The listing builds one solid part. Answer for the finished solid, in the listing's coordinates (mm). Coordinates: 2 decimals unless noted, no trailing zeros. Order: outer loops, then holes, each group sorted by start corner. A loop starts at its lowest first (then second) coordinate and runs counter-clockwise, first axis right, second up.
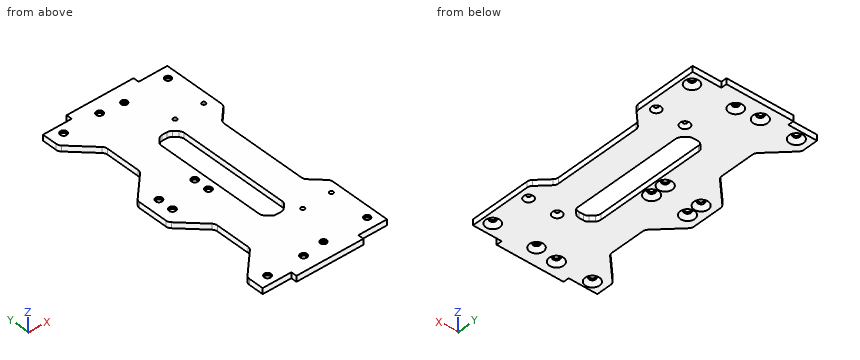
from build123d import *

# Parameters (mm, degrees)
SKETCH_1_W          = 65
SKETCH_1_H          = 129
SKETCH_1_W_2        = 35
SKETCH_1_H_2        = 6
EXTRUDE_1_DEPTH     = 3
SKETCH_2_R          = 1.75
CUT_EXTRUDE_1_DEPTH = 10
CHAMFER_1_SIZE      = 2
SKETCH_3_R          = 1
CUT_EXTRUDE_2_DEPTH = 10
CHAMFER_2_SIZE      = 1.5
CUT_EXTRUDE_3_DEPTH = 10
FILLET_1_R          = 3
CUT_EXTRUDE_4_DEPTH = 22
FILLET_2_R          = 3
SKETCH_6_R          = 1.625
CUT_EXTRUDE_5_DEPTH = 22
CHAMFER_3_SIZE      = 2
CUT_EXTRUDE_6_DEPTH = 22
FILLET_3_R          = 3


with BuildPart() as part:
    # Эскиз1 → Бобышка-Вытянуть1 (new body)
    with BuildSketch(Plane.XY):
        Rectangle(SKETCH_1_W, SKETCH_1_H)
        with Locations((0, 64.5)):
            Rectangle(SKETCH_1_W_2, SKETCH_1_H_2)
        with Locations((0, -64.5)):
            Rectangle(SKETCH_1_W_2, SKETCH_1_H_2)
    extrude(amount=EXTRUDE_1_DEPTH)

    # Эскиз2 → Вырез-Вытянуть1 (cut)
    with BuildSketch(Plane.XY.offset(3)):
        with Locations((-25.8, 59.9)):
            Circle(SKETCH_2_R)
        with Locations((-7, 59.9)):
            Circle(SKETCH_2_R)
        with Locations((-25.8, 4)):
            Circle(SKETCH_2_R)
        with Locations((-7, 4)):
            Circle(SKETCH_2_R)
        with Locations((-7, -4)):
            Circle(SKETCH_2_R)
        with Locations((-25.8, -4)):
            Circle(SKETCH_2_R)
        with Locations((-7, -59.9)):
            Circle(SKETCH_2_R)
        with Locations((-25.8, -59.9)):
            Circle(SKETCH_2_R)
    extrude(amount=-CUT_EXTRUDE_1_DEPTH, mode=Mode.SUBTRACT)

    # Фаска1
    chamfer_1_edges = [part.edges().sort_by_distance(p)[0] for p in [
        (-8.75, 4, 0),
        (-27.55, 4, 0),
        (-8.75, -4, 0),
        (-8.75, 59.9, 0),
        (-27.55, -59.9, 0),
        (-8.75, -59.9, 0),
        (-27.55, -4, 0),
        (-27.55, 59.9, 0),
    ]]
    chamfer(chamfer_1_edges, length=CHAMFER_1_SIZE)

    # Эскиз3 → Вырез-Вытянуть2 (cut)
    with BuildSketch(Plane(origin=(0, 0, 0), x_dir=(-1, 0, 0), z_dir=(0, 0, -1))):
        with Locations((-27.5, 37.5)):
            Circle(SKETCH_3_R)
        with Locations((-12.5, 37.5)):
            Circle(SKETCH_3_R)
        with Locations((-27.5, -37.5)):
            Circle(SKETCH_3_R)
        with Locations((-12.5, -37.5)):
            Circle(SKETCH_3_R)
    extrude(amount=-CUT_EXTRUDE_2_DEPTH, mode=Mode.SUBTRACT)

    # Фаска2
    chamfer_2_edges = [part.edges().sort_by_distance(p)[0] for p in [
        (13.5, 37.5, 0),
        (28.5, -37.5, 0),
        (13.5, -37.5, 0),
        (28.5, 37.5, 0),
    ]]
    chamfer(chamfer_2_edges, length=CHAMFER_2_SIZE)

    # Эскиз4 → Вырез-Вытянуть3 (cut)
    with BuildSketch(Plane(origin=(0, 0, 0), x_dir=(-1, 0, 0), z_dir=(0, 0, -1))):
        Polygon((32.5, 55.5), (19.5, 42.5), (19.5, 22), (32.5, 9), (37.771171481, 9), (37.771171481, 55.5), align=None)
        Polygon((37.771171481, -9), (32.5, -9), (19.5, -22), (19.5, -42.5), (32.5, -55.5), (37.771171481, -55.5), align=None)
    extrude(amount=-CUT_EXTRUDE_3_DEPTH, mode=Mode.SUBTRACT)

    # Скругление1
    fillet_1_edges = [part.edges().sort_by_distance(p)[0] for p in [
        (-32.5, 55.5, 1.5),
        (-32.5, 9, 1.5),
        (-19.5, 22, 1.5),
        (-19.5, 42.5, 1.5),
        (-32.5, -55.5, 1.5),
        (-19.5, -42.5, 1.5),
        (-19.5, -22, 1.5),
        (-32.5, -9, 1.5),
    ]]
    fillet(fillet_1_edges, radius=FILLET_1_R)

    # Эскиз5 → Вырез-Вытянуть4 (cut)
    with BuildSketch(Plane.XY.offset(3)):
        Polygon((1, 33.5), (6, 33.5), (9.5, 30), (9.5, -30), (6, -33.5), (1, -33.5), (-2.5, -30), (-2.5, 30), align=None)
    extrude(amount=-CUT_EXTRUDE_4_DEPTH, mode=Mode.SUBTRACT)

    # Скругление2
    fillet_2_edges = [part.edges().sort_by_distance(p)[0] for p in [
        (-2.5, 30, 1.5),
        (1, 33.5, 1.5),
        (6, 33.5, 1.5),
        (9.5, 30, 1.5),
        (9.5, -30, 1.5),
        (6, -33.5, 1.5),
        (1, -33.5, 1.5),
        (-2.5, -30, 1.5),
    ]]
    fillet(fillet_2_edges, radius=FILLET_2_R)

    # Эскиз6 → Вырез-Вытянуть5 (cut)
    with BuildSketch(Plane(origin=(0, 0, 0), x_dir=(-1, 0, 0), z_dir=(0, 0, -1))):
        with Locations((-27.5, 58.5)):
            Circle(SKETCH_6_R)
        with Locations((-4.64, 58.5)):
            Circle(SKETCH_6_R)
        with Locations(Location((-4.64, -58.5, 0), (0, 0, 180))):
            Circle(SKETCH_6_R)
        with Locations(Location((-27.5, -58.5, 0), (0, 0, 180))):
            Circle(SKETCH_6_R)
    extrude(amount=-CUT_EXTRUDE_5_DEPTH, mode=Mode.SUBTRACT)

    # Фаска3
    chamfer_3_edges = [part.edges().sort_by_distance(p)[0] for p in [
        (25.875, -58.5, 0),
        (3.015, -58.5, 0),
        (6.265, 58.5, 0),
        (29.125, 58.5, 0),
    ]]
    chamfer(chamfer_3_edges, length=CHAMFER_3_SIZE)

    # Эскиз7 → Вырез-Вытянуть6 (cut)
    with BuildSketch(Plane(origin=(0, 0, 0), x_dir=(-1, 0, 0), z_dir=(0, 0, -1))):
        Polygon((-32.5, 31.5), (-25, 24), (-25, -24), (-32.5, -31.5), (-45.278414839, -31.5), (-45.278414839, 31.5), align=None)
    extrude(amount=-CUT_EXTRUDE_6_DEPTH, mode=Mode.SUBTRACT)

    # Скругление3
    fillet_3_edges = [part.edges().sort_by_distance(p)[0] for p in [
        (32.5, 31.5, 1.5),
        (25, 24, 1.5),
        (25, -24, 1.5),
        (32.5, -31.5, 1.5),
    ]]
    fillet(fillet_3_edges, radius=FILLET_3_R)


solid = part.part
1) Each of these flat-tipped pins is pushed along its axis until it touches: P1, Ø1, axis at y = -10, z = 1, coming from the +X side; P2, Ø1.5, axis at y = 31.5, z = 2, coming from the -X side; P3, Ø1.5, axis at y = 66.5, z = 2, coming from the +X side. Where does it stop, or does it pass through?
2) Section B-B (y = 15) is taken. Give the vertices of the cut face in (x, z), then the cut area to 4 significant figures.
3) Consider L1, parallel to Y at x = 4.5, z = 2.35; L2, parallel to Y at x = -7, z = 2.55; L3, parallel to X at y = -58.5, z = 2.7 (3 decimals). Determine where each line is inside the solid, lowest interval first.
4) Section D-D (z = 0.7) is taken. Give the number of separate pieces and of enclosed holes in the cut face, then the cut area to 3 significant figures.
5) Section C-C (y = 53) is taken. Give the vertices of the cut face in (x, z).
6) Section A-A (x = -7) is taken. Give the vertices of the cut face in (y, z), then the cut area to 3 significant figures.
Filled sheet:
1. P1: stops at x = 25
1. P2: stops at x = -19.5
1. P3: stops at x = 17.5
2. outline: (-26.5, 0) - (-2.5, 0) - (-2.5, 3) - (-26.5, 3) - close; (9.5, 0) - (25, 0) - (25, 3) - (9.5, 3) - close
2. area: 118.5 mm2
3. L1: y = -67.5 to -60.12, -56.88 to -33.5, 33.5 to 56.88, 60.12 to 67.5
3. L2: y = -67.5 to -61.65, -58.15 to -5.75, -2.25 to 2.25, 5.75 to 58.15, 61.65 to 67.5
3. L3: x = -32.5 to -26.85, -24.75 to -8.05, -5.95 to 3.015, 6.265 to 25.875, 29.125 to 32.5
4. separate pieces: 1
4. enclosed holes: 17
4. area: 6,150 mm2
5. outline: (-30, 0) - (32.5, 0) - (32.5, 3) - (-30, 3) - close
6. outline: (-67.5, 0) - (-63.65, 0) - (-61.65, 2) - (-61.65, 3) - (-67.5, 3) - close; (-58.15, 2) - (-56.15, 0) - (-7.75, 0) - (-5.75, 2) - (-5.75, 3) - (-58.15, 3) - close; (-2.25, 2) - (-0.25, 0) - (0.25, 0) - (2.25, 2) - (2.25, 3) - (-2.25, 3) - close; (5.75, 2) - (7.75, 0) - (56.15, 0) - (58.15, 2) - (58.15, 3) - (5.75, 3) - close; (61.65, 2) - (63.65, 0) - (67.5, 0) - (67.5, 3) - (61.65, 3) - close
6. area: 347 mm2
